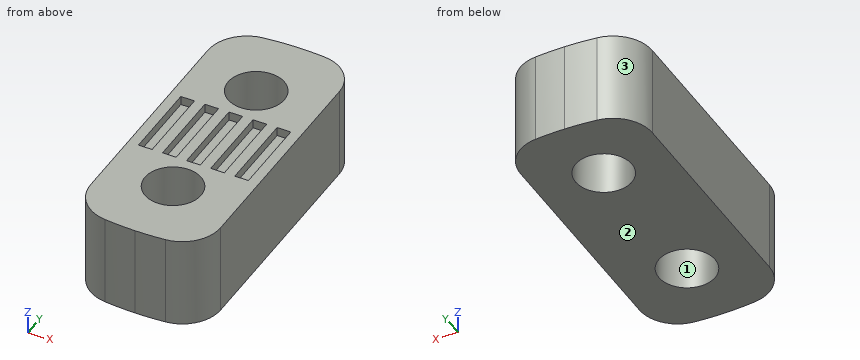
```python
from build123d import *

# Parameters (mm, degrees)
SKETCH1_R           = 2.15
BOSS_EXTRUDE1_DEPTH = 7
SKETCH4_W           = 1.04528
SKETCH4_H           = 6.1088
CUT_EXTRUDE2_DEPTH  = 0.68


with BuildPart() as part:
    # Sketch1 → Boss-Extrude1 (new body)
    with BuildSketch(Plane.XY):
        with BuildLine():
            Line((-5, 14.434422223), (-5, -2.434422223))
            ThreePointArc((-5, -2.434422223), (-4.239496508, -4.429977284), (-2.343767283, -5.413245441))
            ThreePointArc((-2.343767283, -5.413245441), (-1.151217334, -5.519255542), (0.045204926, -5.563834645))
            ThreePointArc((0.045204926, -5.563834645), (1.187062084, -5.549004877), (2.326819369, -5.478216303))
            ThreePointArc((2.326819369, -5.478216303), (4.230533554, -4.540680035), (5, -2.563049296))
            Line((5, -2.563049296), (5, 14.563049296))
            ThreePointArc((5, 14.563049296), (4.230533554, 16.540680035), (2.326819369, 17.478216303))
            ThreePointArc((2.326819369, 17.478216303), (1.187062084, 17.549004877), (0.045204926, 17.563834645))
            ThreePointArc((0.045204926, 17.563834645), (-1.151217334, 17.519255542), (-2.343767283, 17.413245441))
            ThreePointArc((-2.343767283, 17.413245441), (-4.239496508, 16.429977284), (-5, 14.434422223))
        make_face()
        Circle(SKETCH1_R, mode=Mode.SUBTRACT)
        with Locations((0, 12)):
            Circle(SKETCH1_R, mode=Mode.SUBTRACT)
    extrude(amount=BOSS_EXTRUDE1_DEPTH)

    # Sketch4 → Cut-Extrude2 (cut)
    with BuildSketch(Plane.XY.offset(7)):
        with Locations((-3.68176, 6)):
            Rectangle(SKETCH4_W, SKETCH4_H)
        with Locations((-1.84088, 6)):
            Rectangle(SKETCH4_W, SKETCH4_H)
        with Locations((0, 6)):
            Rectangle(SKETCH4_W, SKETCH4_H)
        with Locations((1.84088, 6)):
            Rectangle(SKETCH4_W, SKETCH4_H)
        with Locations((3.68176, 6)):
            Rectangle(SKETCH4_W, SKETCH4_H)
    extrude(amount=-CUT_EXTRUDE2_DEPTH, mode=Mode.SUBTRACT)


solid = part.part
```
Here's how the part is built. I have some questions about the finished solid (model axes, mm). Face numbers are marked on the shaded views. Coordinates: 2 decimals unless noted, no trailing zeros. Order: outer loops, then holes, each group sorted by start corner. A loop starts at its lowest first (then second) coordinate and runs counter-clockwise, first axis right, second up.
1) Imagine slicing it at C-C on x = -3.5. List the corners of the cut face in (y, z) for me, and give its area (3 significant figures).
2) Imagine slicing it at B-B on z = 3.5. State how many separate pieces and enclosed holes the cut face has, and give its area (3 significant figures).
3) Imagine slicing it at A-A on y = 0. List the corners of the cut face in (x, z) for me, and give its area (3 significant figures).
4) Will these pins go through, and if not, where does the flat tip stop? pin 1 (0.5 mm diameter, centred on x = 0, y = 6, fed in from +Z); pin 2 (0.5 mm diameter, centred on x = -2, z = 7, fed in from +Y); pin 3 (0.5 mm diameter, centred on x = -4, z = 6.5, fed in from -Y).
5) I need wall thicknesses on line 1 (Y direction, x = 0, z = 3); line 2 (X direction, y = 7.5, z = 6.5); line 3 (Y direction, x = 1.75, z = 6.5). Which ranges of each line are inside material? Lowest first, please.
6) We'd pull the mould along Y, two halves only. Please class the marked faces 1, 2 and 3: +Y half, -Y half, draft (parallel to the pull), parting line (faces both ways), or undercut.
Response values:
1. outline: (-5.03, 0) - (17.03, 0) - (17.03, 7) - (9.05, 7) - (9.05, 6.32) - (2.95, 6.32) - (2.95, 7) - (-5.03, 7) - close
1. area: 150 mm2
2. separate pieces: 1
2. enclosed holes: 2
2. area: 193 mm2
3. outline: (-5, 0) - (-2.15, 0) - (-2.15, 7) - (-5, 7) - close; (2.15, 0) - (5, 0) - (5, 7) - (2.15, 7) - close
3. area: 39.9 mm2
4. pin 1: stops at z = 6.32
4. pin 2: stops at y = 17.47
4. pin 3: stops at y = -4.87
5. line 1: y = -5.56 to -2.15, 2.15 to 9.85, 14.15 to 17.56
5. line 2: x = -5 to -4.2, -3.16 to -2.36, -1.32 to -0.52, 0.52 to 1.32, 2.36 to 3.16, 4.2 to 5
5. line 3: y = -5.52 to -1.25, 1.25 to 2.95, 9.05 to 10.75, 13.25 to 17.52
6. face 1: undercut
6. face 2: draft
6. face 3: +Y half
